Could you check a few things on this model? Use its own coordinates, in mm. A direction names the side the tool comes from. Give positions to 0.01 mm unless a question says otherwise; leave off trailing zeros. Order: outer loops, then holes, each group sorted by start corner. A loop starts at its lowest first (then second) coordinate and runs counter-clockwise, first axis right, second up.
Autodesk Inventor part; units mm, degrees
ref_plane "YZ Plane" through (0, 0, 0) normal (1, 0, 0) x (0, 1, 0)
ref_plane "XZ Plane" through (0, 0, 0) normal (0, 1, 0) x (-1, 0, 0)
ref_plane "XY Plane" through (0, 0, 0) normal (0, 0, 1) x (1, 0, 0)
sketch "Sketch1" plane through (0, 0, 0) normal (0, 0, 1) x (1, 0, 0)
  line L0 (0, 0) -> (64.77, 0)
  line L1 (64.77, 0) -> (64.77, 175.26)
  line L2 (64.77, 175.26) -> (0, 175.26)
  line L3 (0, 175.26) -> (0, 0)
  dimension "d0" = 64.77
  dimension "d1" = 175.26
extrude "Extrusion1" add sketch "Sketch1" along normal blind 50.8
shell "Shell1" thickness 1.5875 outward yes removed faces 1 at (21.59, 116.84, 0)
sketch "Sketch2" plane through (0, 175.26, 0) normal (0, -1, 0) x (1, 0, 0)
  line L0 (64.77, 50.8) -> (0, 50.8)
  line L1 (64.77, 50.8) -> (0, 50.8)
  line L2 (0, 50.8) -> (0, 41.275)
  line L3 (0, 41.275) -> (64.77, 41.275)
  line L4 (64.77, 41.275) -> (64.77, 50.8)
  line L5 (60.706, 41.275) -> (46.482, 41.275)
  line L6 (46.482, 41.275) -> (46.482, 36.5125)
  line L7 (46.482, 36.5125) -> (60.706, 36.5125)
  line L8 (60.706, 36.5125) -> (60.706, 41.275)
  line L9 (25.4, 41.275) -> (6.35, 41.275)
  line L10 (6.35, 41.275) -> (6.35, 32.385)
  line L11 (6.35, 32.385) -> (25.4, 32.385)
  line L12 (25.4, 32.385) -> (25.4, 41.275)
  point P0 (0, 0)
  point P1 (6.35, 41.275)
  dimension "d5" = 9.525
  dimension "d6" = 64.77
  dimension "d7" = 4.7625
  dimension "d8" = 14.224
  dimension "d9" = 18.288
  dimension "d10" = 19.05
  dimension "d11" = 25.4
  dimension "d12" = 8.89
sketch "Sketch4" plane through (0, 0, 0) normal (0, 1, 0) x (1, 0, 0)
  line L0 (0, 0) -> (0, -50.8)
  line L1 (0, -50.8) -> (64.77, -50.8)
  line L2 (64.77, -50.8) -> (64.77, -41.275)
  line L3 (64.77, -41.275) -> (0, -41.275)
  line L4 (0, -41.275) -> (0, -50.8)
  line L5 (37.7825, -41.275) -> (60.0075, -41.275)
  line L6 (60.0075, -41.275) -> (60.0075, -25.4)
  line L7 (60.0075, -25.4) -> (37.7825, -25.4)
  line L8 (37.7825, -25.4) -> (37.7825, -41.275)
  line L9 (20.6375, -41.275) -> (33.3375, -41.275)
  line L10 (33.3375, -41.275) -> (33.3375, -34.925)
  line L11 (33.3375, -34.925) -> (20.6375, -34.925)
  line L12 (20.6375, -34.925) -> (20.6375, -41.275)
  dimension "d13" = 9.525
  dimension "d14" = 64.77
  dimension "d15" = 22.225
  dimension "d16" = 15.875
  dimension "d17" = 26.9875
  dimension "d18" = 12.7
  dimension "d19" = 6.35
  dimension "d20" = 33.3375
sketch "Sketch5" plane through (0, 0, 0) normal (1, 0, 0) x (0, 0, -1)
  line L0 (-50.8, 175.26) -> (-50.8, 0)
  line L1 (-50.8, 175.26) -> (-41.275, 175.26)
  line L2 (-41.275, 175.26) -> (-41.275, 0)
  line L3 (-41.275, 0) -> (-50.8, 0)
  line L4 (-50.8, 0) -> (-50.8, 175.26)
  line L5 (-41.275, 139.192) -> (-32.385, 139.192)
  line L6 (-32.385, 139.192) -> (-32.385, 121.412)
  line L7 (-32.385, 121.412) -> (-41.275, 121.412)
  line L8 (-41.275, 121.412) -> (-41.275, 139.192)
  point P0 (0, 0)
  dimension "d21" = 9.525
  dimension "d22" = 175.26
  dimension "d23" = 17.78
  dimension "d24" = 8.89
  dimension "d25" = 53.848
extrude "Extrusion2" cut sketch "Sketch5" along normal mid plane 171.45 contours L5 L6 L7 L2
extrude "Extrusion3" cut sketch "Sketch2" against normal blind 171.45 contours L8 L7 L6 L3 | L3 L12 L11 L10
extrude "Extrusion4" cut sketch "Sketch4" against normal blind 171.45 contours L12 L11 L10 L3 | L8 L7 L6 L3
sketch "Sketch6" plane through (-1.5875, -1.5875, 0) normal (-1, 0, 0) x (0, 0, 1)
  line L0 (0, 0) -> (52.3875, 0)
  line L1 (0, 0) -> (0, 25.4)
  line L2 (0, 176.8475) -> (0, 1.5875)
  line L3 (0, 25.4) -> (26.1938, 58.1347)
  line L4 (26.1938, 58.1347) -> (26.1938, 178.435)
  line L5 (0, 178.435) -> (52.3875, 178.435)
  line L6 (0, 178.435) -> (0, 25.4)
  dimension "d32" = 25.4
extrude "Extrusion5" cut sketch "Sketch6" against normal blind 171.45
sketch "Sketch7" plane through (-1.5875, -1.5875, 0) normal (0, -1, 0) x (1, 0, 0)
  circle A0 centre (5.207, 18.4912) radius 2.25
  line L0 (0, 0) -> (0, 52.3875)
  line L1 (0, 0) -> (67.945, 0)
  circle A1 centre (40.207, 18.4912) radius 2.25
  point P0 (1.5875, 0)
  dimension "d35" = 4.5
  dimension "d36" = 5.207
  dimension "d37" = 18.4912
  dimension "d38" = 4.5
  dimension "d39" = 35
extrude "Extrusion6" cut sketch "Sketch7" against normal blind 171.45
sketch "Sketch8" plane through (-1.5875, -1.5875, 0) normal (0, -1, 0) x (1, 0, 0)
  circle A0 centre (22.707, 26.4912) radius 5.5
  circle A1 centre (5.207, 18.4912) radius 2.25
  point P0 (1.5875, 0)
  dimension "d42" = 11
  dimension "d43" = 8
  dimension "d44" = 17.5
extrude "Extrusion7" cut sketch "Sketch8" against normal blind 10 contours A0
sketch "Sketch9" plane through (66.3575, -1.5875, 52.3875) normal (1, 0, 0) x (0, 0, -1)
  circle A0 centre (37.3875, 5) radius 1.5
  circle A1 centre (37.3875, 34.5) radius 1.5
  line L0 (52.3875, 0) -> (0, 0)
  line L1 (52.3875, 0) -> (52.3875, 25.4)
  point P0 (52.3875, 1.5875)
  dimension "d47" = 3
  dimension "d48" = 3
  dimension "d49" = 29.5
  dimension "d50" = 5
  dimension "d51" = 15
  dimension "d52" = 15
extrude "Extrusion8" cut sketch "Sketch9" against normal blind 10
properties part number "_3DPrint"
Item 1: For faces 4 (the cylindrical face through (16.755, -0.805, 23.145)), 5 (the cylindrical face through (65.57, 3.48, 16.5)), 6 (the flat face through (32, 0, 25)), which set-ups out of +Z, -Z, +X, -X, +Y, -Y let a thin tool reach every point of the face, with its end or its side?
Findings:
face 4: -Y
face 5: +X
face 6: -Z
Item 2: Please list where these lines run through material, in increasing order: line 1 along Y through (x, z) = (65.65, 15); line 2 along X through (y, z) = (49, 50.5); line 3 along Y through (x, z) = (3.5, 29).
Findings:
line 1: y = -1.59 to 1.91, 4.91 to 31.41, 34.41 to 42.56
line 2: x = -1.59 to 0, 64.77 to 66.36
line 3: y = -1.59 to 0, 175.26 to 176.85
Item 3: Imagine slicing it at C-C on z = 48.5. List the corners of the cut face in (x, y) for me, then the cut area to 3 significant figures.
Findings:
outline: (-1.59, -1.59) - (66.36, -1.59) - (66.36, 176.85) - (-1.59, 176.85) - close; hole (0, 0) - (64.77, 0) - (64.77, 175.26) - (0, 175.26) - close
area: 772 mm2
Item 4: For pin 1 (19.5 mm diameter, centred on x = 23, y = 111, fed in from -Z); pin 2 (0.5 mm diameter, centred on x = -0.5, y = 130, fed in from -Z); pin 3 (2 mm diameter, centred on x = 26, z = 22, fed in from +Y), each with a flat end and sliding along its axis, tell me the tip position at first contact or that it passes through.
Findings:
pin 1: stops at z = 50.8
pin 2: stops at z = 26.19
pin 3: stops at y = 0
Item 5: We'd pull the mould along Z, two halves only. Please class faces 1 (the cylindrical face through (65.57, 32.98, 16.5)), 2 (the flat face through (30, -1, 0)), 3 (the flat face through (66.358, 67, 32)): +Z half, -Z half, draft (parallel to the pull), parting line (faces both ways), or undercut.
Findings:
face 1: undercut
face 2: -Z half
face 3: draft
Item 6: Imagine slicing it at A-A on z = 39. Give the number of separate pieces and of enclosed holes in the cut face, then the cut area to 3 significant figures.
Findings:
separate pieces: 6
enclosed holes: 0
area: 607 mm2
Item 7: Imagine slicing it at D-D on y = 79. List the corners of the cut face in (x, z) for me, then the cut area to 3 significant figures.
Findings:
outline: (-1.59, 26.19) - (0, 26.19) - (0, 50.8) - (64.77, 50.8) - (64.77, 26.19) - (66.36, 26.19) - (66.36, 52.39) - (-1.59, 52.39) - close
area: 186 mm2
Item 8: Imagine slicing it at B-B on x = 52.5. List the corners of the cut face in (y, z) for me (1 decimal).
Findings:
outline: (-1.6, 0) - (0, 0) - (0, 25.4) - (-1.6, 25.4) - close; (-1.6, 41.3) - (0, 41.3) - (0, 50.8) - (175.3, 50.8) - (175.3, 41.3) - (176.8, 41.3) - (176.8, 52.4) - (-1.6, 52.4) - close; (175.3, 26.2) - (176.8, 26.2) - (176.8, 36.5) - (175.3, 36.5) - close
